from build123d import *

# Parameters (mm, degrees)
SKETCH2_W           = 25.146
SKETCH2_H           = 177.8
BOSS_EXTRUDE1_DEPTH = 5.08
SKETCH4_W           = 25.146
SKETCH4_H           = 25.4
CUT_EXTRUDE2_DEPTH  = 2.54
BOSS_EXTRUDE2_DEPTH = 12.7
SKETCH6_R           = 3
CUT_EXTRUDE3_DEPTH  = 146.707735218
BOSS_EXTRUDE3_DEPTH = 7.62
SKETCH9_R           = 1.5
CUT_EXTRUDE4_DEPTH  = 10.668


with BuildPart() as part:
    # Sketch2 → Boss-Extrude1 (new body)
    with BuildSketch(Plane(origin=(0, 0, 0), x_dir=(1, 0, 0), z_dir=(0, 1, 0))):
        with Locations((1.939834286, -54.988822857)):
            Rectangle(SKETCH2_W, SKETCH2_H)
    extrude(amount=BOSS_EXTRUDE1_DEPTH)

    # Sketch4 → Cut-Extrude2 (cut)
    with BuildSketch(Plane.XZ):
        with Locations((1.939834286, 131.188822857)):
            Rectangle(SKETCH4_W, SKETCH4_H)
    extrude(amount=-CUT_EXTRUDE2_DEPTH, mode=Mode.SUBTRACT)

    # Sketch5 → Boss-Extrude2 (add)
    with BuildSketch(Plane(origin=(0, 5.08, 0), x_dir=(1, 0, 0), z_dir=(0, 1, 0))):
        with BuildLine():
            Line((14.512834286, 19.170963767), (14.512834286, 15.062455759))
            ThreePointArc((14.512834286, 15.062455759), (5.213589162, 8.191698096), (-0.187237198, -2.031527684))
            Line((-0.187237198, -2.031527684), (-3.867414596, -1.045427123))
            ThreePointArc((-3.867414596, -1.045427123), (2.870150259, 11.292575602), (14.512834286, 19.170963767))
        make_face()
        with BuildLine():
            Line((14.512834286, -32.584101473), (14.512834286, -36.692609481))
            ThreePointArc((14.512834286, -36.692609481), (2.870150259, -28.814221316), (-3.867414596, -16.476218592))
            Line((-3.867414596, -16.476218592), (-0.187237198, -15.49011803))
            ThreePointArc((-0.187237198, -15.49011803), (5.213589162, -25.713343811), (14.512834286, -32.584101473))
        make_face()
    extrude(amount=BOSS_EXTRUDE2_DEPTH)

    # Sketch6 → Cut-Extrude3 (cut, through all)
    with BuildSketch(Plane.XZ):
        with Locations(Location((2.066834286, 8.760822857, 0), (0, 0, 270))):
            Circle(SKETCH6_R)
    extrude(amount=-CUT_EXTRUDE3_DEPTH, mode=Mode.SUBTRACT)

    # Sketch8 → Boss-Extrude3 (add)
    with BuildSketch(Plane(origin=(0, 5.08, 0), x_dir=(1, 0, 0), z_dir=(0, 1, 0))):
        Polygon((18.409653056, -90.331413744), (18.409653056, -87.791413744), (10.639653056, -87.791413744), (10.639653056, -96.071413744), (18.409653056, -96.071413744), (18.409653056, -93.531413744), (11.909653056, -93.531413744), (11.909653056, -90.331413744), align=None)
    extrude(amount=BOSS_EXTRUDE3_DEPTH)

    # Sketch9 → Cut-Extrude4 (cut)
    with BuildSketch(Plane.XY.offset(96.071413744)):
        with Locations((14.195653056, 10.414)):
            Circle(SKETCH9_R)
    extrude(amount=-CUT_EXTRUDE4_DEPTH, mode=Mode.SUBTRACT)


solid = part.part
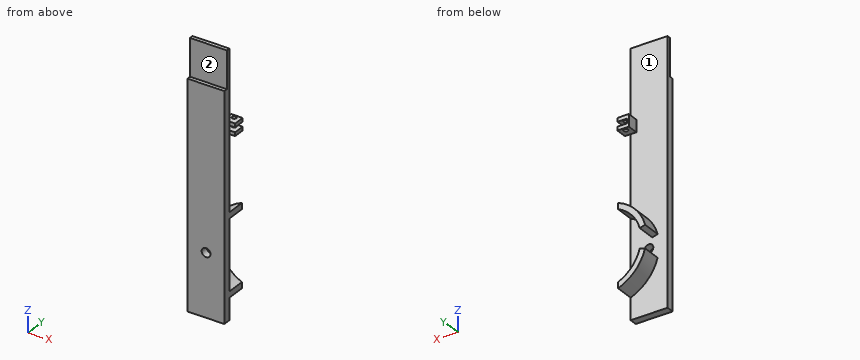
Work out the finished part from the listing and answer in its coordinate system (mm). Face numbers are marked on the shaded views. Give positions to 0.01 mm unless a question says otherwise; leave off trailing zeros. Order: outer loops, then holes, each group sorted by start corner. A loop starts at its lowest first (then second) coordinate and runs counter-clockwise, first axis right, second up. Notation, with made-up numbers: (56, 82.5) -> (87, 82.5) arc R21 ccw to (87, 105.5) -> close; hole circle Ø11 at (58, 0.25). An arc over 180 degrees is marked (long way). Answer as a JSON object with one key per item and string values. Group by question number.
1. Section D-D on x = 8.75 is taken. Determine the outline of the cut face in (y, z).
2. Consider line 1 along Z through (x, y) = (11.75, 7); line 2 along Z through (x, y) = (10.75, 9.25); line 3 along Y through (x, z) = (-4.5, -24.5). Determine where each line is inside the solid, lowest interval first. Write a range as [from, to].
3. Section C-C on z = 64 is taken. Determine the outline of the cut face in (x, y), plus the area to 3 significant figures.
4. Section B-B on x = -5.5 is taken. Determine the outline of the cut face in (y, z).
5. Flat-ended cylindrical pins translate along their axes: pin 1 Ø8.5 at (x, y) = (15.5, 10) entering from +Z; pin 2 Ø4 at (y, z) = (11.5, 37.5) entering from -X; pin 3 Ø2.5 at (x, z) = (14, 91) entering from +Y; pin 4 Ø1.5 at (y, z) = (6.5, 80.5) entering from +X. Find the tip coordinate at first contact, or state that the pin passes through.
6. The mould has two halves that part along Z. Classify the marked faces 1 and 2: released by +Z, released by -Z, zero draft, split by the parting line, or undercut.
7. Section A-A on y = 16 is taken. Determine the outline of the cut face in (x, z), plus the area to 3 significant figures.
Result sheet:
{
 "1": {"outline": "(0, -33.91) -> (5.08, -33.91) -> (5.08, -16.28) -> (17.78, -16.28) -> (17.78, -11.59) -> (5.08, -11.59) -> (5.08, 29.12) -> (17.78, 29.12) -> (17.78, 33.8) -> (5.08, 33.8) -> (5.08, 143.89) -> (2.54, 143.89) -> (2.54, 118.49) -> (0, 118.49) -> close"},
 "2": {"line 1": "z = [-17.98, -13.65], [31.17, 35.5], [87.79, 96.07]", "line 2": "z = [-17.46, -13.03], [30.56, 34.98], [87.79, 96.07]", "line 3": "y = [0, 5.08]"},
 "3": {"outline": "(-10.63, 0) -> (14.51, 0) -> (14.51, 5.08) -> (-10.63, 5.08) -> close", "area": "128 mm^2"},
 "4": {"outline": "(0, -33.91) -> (5.08, -33.91) -> (5.08, 143.89) -> (2.54, 143.89) -> (2.54, 118.49) -> (0, 118.49) -> close"},
 "5": {"pin 1": "stops at z = 96.07", "pin 2": "stops at x = 11.75", "pin 3": "stops at y = 12.7", "pin 4": "passes through"},
 "6": {"face 1": "undercut", "face 2": "zero draft"},
 "7": {"outline": "(-3.87, 1.05) arc R29.81 ccw to (14.51, -19.17) -> (14.51, -15.06) arc R26 cw to (-0.19, 2.03) -> close; (-3.87, 16.48) -> (-0.19, 15.49) arc R26 cw to (14.51, 32.58) -> (14.51, 36.69) arc R29.81 ccw to start", "area": "197 mm^2"}
}
